```python
from build123d import *

# Parameters (mm, degrees)
SKETCH1_W           = 198
SKETCH1_H           = 40
BOSS_EXTRUDE1_DEPTH = 3
BOSS_EXTRUDE2_DEPTH = 198


with BuildPart() as part:
    # Sketch1 → Boss-Extrude1 (new body)
    with BuildSketch(Plane(origin=(0, 0, 0), x_dir=(1, 0, 0), z_dir=(0, 1, 0))):
        Rectangle(SKETCH1_W, SKETCH1_H)
    extrude(amount=BOSS_EXTRUDE1_DEPTH)

    # Sketch2 → Boss-Extrude2 (add)
    with BuildSketch(Plane(origin=(-99, 0, 2.522926574), x_dir=(0, 0, 1), z_dir=(-1, 0, 0))):
        Polygon((0, 0), (0, -14.161533961), (14.925088272, 0), align=None)
    extrude(amount=-BOSS_EXTRUDE2_DEPTH)


solid = part.part
```
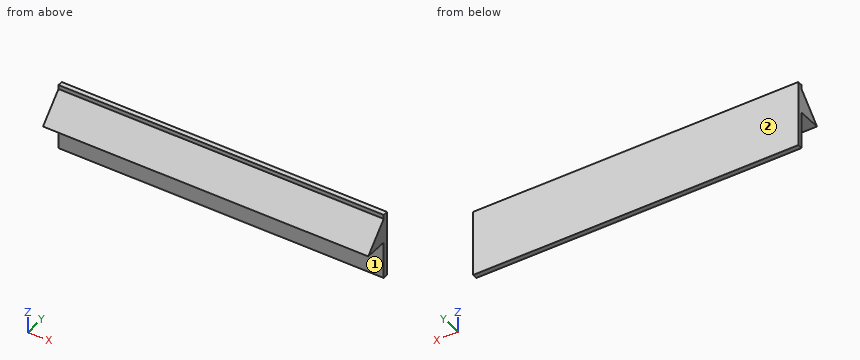
Could you check a few things on this model? Use its own coordinates, in mm. Face numbers are marked on the shaded views. A direction names the side the tool comes from. Round coordinates to 2 decimals unless told otherwise and drop trailing zeros. Order: outer loops, then holes, each group sorted by start corner. A loop starts at its lowest first (then second) coordinate and runs counter-clockwise, first axis right, second up. Notation, with made-up numbers: M 32.5,22 L 70.5,22 A6 cw 70.5,30 Z; hole C -14.5,62 d5. An arc over 180 degrees is marked long. One line per question, with ' | ' between items. Start each with the question number.
(1) Please list where these lines run through material, in increasing order: line 1 along Y through (x, z) = (-6, -12.5); line 2 along Y through (x, z) = (-30.5, 6.5); line 3 along Z through (x, y) = (-35, -12.25).
(2) Suppose I cut it at C-C on y = -12. List the corners of the cut face in (x, z) for me, then the cut area to 3 significant figures.
(3) For P1, Ø3, axis at x = -52, y = -6, coming from the -Z side; P2, Ø1.3, axis at x = 8, z = 19, coming from the -Y side; P3, Ø2, axis at x = 35, y = -10.5, coming from the +Z side, each with a flat end and sliding along its axis, tell me the tip position at first contact or that it passes through.
(4) Suppose I cut it at A-A on x = -11.5. List the corners of the cut face in (y, z) for me.
(5) Suppose I cut it at B-B on z = -6. List the corners of the cut face in (x, y) for me.
(6) For the marked faces 1 and 2, which set-ups out of +Z, -Z, +X, -X, +Y, -Y let a thin tool reach every point of the face, with its end or its side?
Geometry results:
1) line 1: 0 to 3 | line 2: -10.39 to 3 | line 3: 2.52 to 4.54
2) outline: M -99,2.52 L 99,2.52 L 99,4.8 L -99,4.8 Z | area: 451 mm²
3) P1: z = 2.52 | P2: y = 0 | P3: z = 7.44
4) outline: M -14.16,2.52 L 0,2.52 L 0,-20 L 3,-20 L 3,20 L 0,20 L 0,17.45 Z
5) outline: M -99,0 L 99,0 L 99,3 L -99,3 Z
6) face 1: -Z, +X, -X, -Y | face 2: +Z, -Z, +X, -X, +Y
